Geometry: final body of the model. Coordinates: model frame, mm. A direction names the side the tool comes from. Give positions to 0.01 mm unless a question says otherwise; leave off trailing zeros. Order: outer loops, then holes, each group sorted by start corner. A loop starts at its lowest first (then second) coordinate and runs counter-clockwise, first axis right, second up. Notation, with made-up numbers: M 69,-9.5 L 112,-9.5 A8 ccw 112,-2.5 Z; hole C 83.25,-6 d9. An arc over 180 degrees is marked long. One line per item, written item: value. Start each with the question number.
```python
from build123d import *

# Parameters (mm, degrees)
BOSS_EXTRUDE1_DEPTH              = 215.9
FILLET1_R                        = 0.254
SKETCH4_W                        = 25.4
SKETCH4_H                        = 25.4
BOSS_EXTRUDE2_DEPTH              = 12.7
FILLET2_R                        = 1.651
F_10_0_1935_DIAMETER_HOLE1_D     = 4.9149
F_10_0_1935_DIAMETER_HOLE1_DEPTH = 23.923415072
F_10_0_1935_DIAMETER_HOLE1_TIP   = 1.476584928


with BuildPart() as part:
    # Sketch3 → Boss-Extrude1 (new body)
    with BuildSketch(Plane.XY):
        with BuildLine():
            Line((-11.049, 12.7), (-3.302, 12.7))
            Line((-3.302, 12.7), (-3.302, 10.328863887))
            Line((-3.302, 10.328863887), (-6.985, 10.328863887))
            ThreePointArc((-6.985, 10.328863887), (-7.454330803, 10.01526707), (-7.344210245, 9.461653642))
            Line((-7.344210245, 9.461653642), (-3.452505379, 5.569948776))
            ThreePointArc((-3.452505379, 5.569948776), (-2.628470073, 5.019345987), (-1.656454155, 4.826))
            Line((-1.656454155, 4.826), (1.656454155, 4.826))
            ThreePointArc((1.656454155, 4.826), (2.628470073, 5.019345987), (3.452505379, 5.569948776))
            Line((3.452505379, 5.569948776), (7.344210245, 9.461653642))
            ThreePointArc((7.344210245, 9.461653642), (7.454330803, 10.01526707), (6.985, 10.328863887))
            Line((6.985, 10.328863887), (3.302, 10.328863887))
            Line((3.302, 10.328863887), (3.302, 12.7))
            Line((3.302, 12.7), (11.049, 12.7))
            ThreePointArc((11.049, 12.7), (12.216433296, 12.216433296), (12.7, 11.049))
            Line((12.7, 11.049), (12.7, 1.651))
            ThreePointArc((12.7, 1.651), (12.216433296, 0.483566704), (11.049, 0))
            Line((11.049, 0), (-11.049, 0))
            ThreePointArc((-11.049, 0), (-12.216433296, 0.483566704), (-12.7, 1.651))
            Line((-12.7, 1.651), (-12.7, 11.049))
            ThreePointArc((-12.7, 11.049), (-12.216433296, 12.216433296), (-11.049, 12.7))
        make_face()
    extrude(amount=BOSS_EXTRUDE1_DEPTH)

    # Fillet1
    fillet1_edges = [part.edges().sort_by_distance(p)[0] for p in [
        (-3.302, 12.7, 107.95),
        (-3.302, 10.328863887, 107.95),
        (3.302, 10.328863887, 107.95),
        (3.302, 12.7, 107.95),
    ]]
    fillet(fillet1_edges, radius=FILLET1_R)

    # Sketch4 → Boss-Extrude2 (add)
    with BuildSketch(Plane(origin=(0, 0, 0), x_dir=(-1, 0, 0), z_dir=(0, 0, -1))):
        Rectangle(SKETCH4_W, SKETCH4_H)
    extrude(amount=BOSS_EXTRUDE2_DEPTH)

    # Fillet2
    fillet2_edges = [part.edges().sort_by_distance(p)[0] for p in [
        (-12.7, 12.7, -6.35),
        (12.7, 12.7, -6.35),
        (-12.7, -12.7, -6.35),
        (12.7, -12.7, -6.35),
    ]]
    fillet(fillet2_edges, radius=FILLET2_R)

    # #10 (0.1935) Diameter Hole1
    with Locations(Plane(origin=(0, 0, -12.7), x_dir=(-1, 0, 0), z_dir=(0, 0, -1))):
        with Locations((-6.35, -6.35), (6.35, -6.35)):
            Hole(F_10_0_1935_DIAMETER_HOLE1_D / 2, depth=F_10_0_1935_DIAMETER_HOLE1_DEPTH)
            with Locations((0, 0, -(F_10_0_1935_DIAMETER_HOLE1_DEPTH + F_10_0_1935_DIAMETER_HOLE1_TIP / 2))):  # 118° drill point
                Cone(0, F_10_0_1935_DIAMETER_HOLE1_D / 2, F_10_0_1935_DIAMETER_HOLE1_TIP, mode=Mode.SUBTRACT)


solid = part.part
```
Q1. Mould query, pull axis X, two halves, no side actions, for faces 4 (the face through (12.7, 7, 103)), 5 (the face through (-12.7, 7, 103)), 6 (the face through (0, 9, 0)). Classes: +X half, -X half, draft (parallel to the pull), parting line (faces both ways), or undercut.
Q2. Set-up query: faces 1 (the face through (0, 0, 106)), 2 (the face through (-5, 12.7, 103)), 3 (the face through (5.37, 7.49, 106.44)). Return all of +Z, -Z, +X, -X, +Y, -Y with unobstructed straight access to the full face (end or side cutting, diameter ignored); none if empty.
Q3. Section query A-A on y = -6.35. Return loops of the section in (x, z).
Q4. Ray query, line 1 along Y through (x, z) = (5.25, 199.5); line 2 along Y through (x, z) = (6.35, -4); line 3 along X through (y, z) = (8.5, 195.5). Return the intervals inside material, ascending. Write a range as [from, to].
Q5. Contact query for flat-ended pins moving along their axis: pin 1 (2.5 mm diameter, centred on x = -4.5, z = 58, fed in from -Y); pin 2 (11.5 mm diameter, centred on x = 5, y = -6, fed in from +Z); pin 3 (1.7 mm diameter, centred on x = -0.5, z = 140.5, fed in from +Y); pin 4 (4 mm diameter, centred on x = 6.35, y = -6.35, fed in from +Z). Output: stop coordinate, or through.
Results below:
1. face 4: +X half
1. face 5: -X half
1. face 6: undercut
2. face 1: +Z, +X, -X, -Y
2. face 2: +Z, -Z, +X, -X, +Y
2. face 3: +Z
3. outline: M -12.7,-12.7 L -8.81,-12.7 L -8.81,0 L -12.7,0 Z; M -3.89,-12.7 L 3.89,-12.7 L 3.89,0 L -3.89,0 Z; M 8.81,-12.7 L 12.7,-12.7 L 12.7,0 L 8.81,0 Z
4. line 1: [0, 7.37], [10.33, 12.7]
4. line 2: [-12.7, -8.81], [-3.89, 12.7]
4. line 3: [-12.7, -6.38], [6.38, 12.7]
5. pin 1: y = 0
5. pin 2: z = 0
5. pin 3: y = 4.83
5. pin 4: through
